Build history of the part. All positions in model axes, mm. Face numbers are marked on the shaded views. A direction names the side the tool comes from. Round coordinates to 2 decimals unless told otherwise and drop trailing zeros. Write each loop counter-clockwise with the first axis right and the second up, starting at its lowest first coordinate (ties: lowest second). Pieces come first, ordered by that corner, then holes. Notation, with made-up numbers: (1.5, 42.5) - (28.5, 42.5) arc R24 ccw to (28.5, 81.5) - close; hole circle Ø3 at (69, 58). An arc over 180 degrees is marked (long way). Write each question's results on one line, items separated by ' | '.
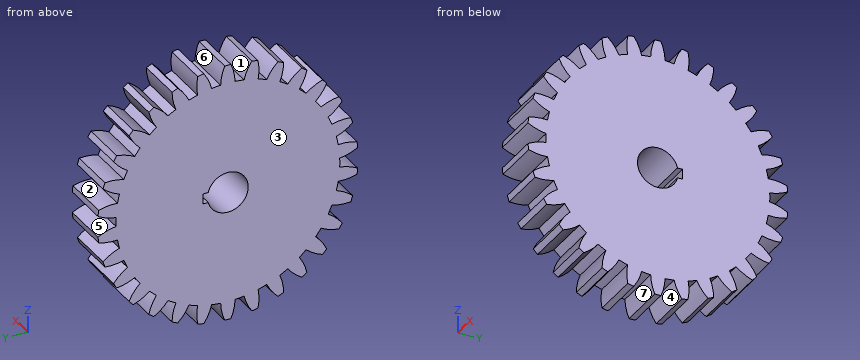
from build123d import *

# Parameters (mm, degrees)
BASPROSKE_W     = 304.8
BASPROSKE_H     = 812.8
TOOTHCUT_DEPTH  = 1190.197510929
TEETHCUTS_COUNT = 30
TEETHCUTS_ANGLE = 348
BORSKE_R        = 127
BORE_DEPTH      = 304.8000508
KEYSKE_W        = 63.5
KEYSKE_H        = 154.8384
KEYWAY_DEPTH    = 304.8000508


with BuildPart() as part:
    # BasProSke → Base-Revolve (revolve)
    with BuildSketch(Plane(origin=(0, 0, 0), x_dir=(1, 0, 0), z_dir=(0, 1, 0)), mode=Mode.PRIVATE) as base_revolve_sk:
        with Locations((152.4, 406.4)):
            Rectangle(BASPROSKE_W, BASPROSKE_H)
    revolve(base_revolve_sk.sketch.rotate(Axis((-10, 0, 0), (1, 0, 0)), 180), axis=Axis((-10, 0, 0), (1, 0, 0)))

    # TooCutSke → ToothCut (cut, through all)
    with BuildSketch(Plane(origin=(0, 0, 0), x_dir=(0, 0, -1), z_dir=(1, 0, 0))):
        with BuildLine():
            ThreePointArc((28.319737367, 697.924400123), (0, 698.49873), (-28.319737367, 697.924400123))
            ThreePointArc((-28.319737367, 697.924400123), (-41.533758507, 755.876600482), (-65.744032335, 810.162238751))
            ThreePointArc((-65.744032335, 810.162238751), (0, 812.8254), (65.744032335, 810.162238751))
            ThreePointArc((65.744032335, 810.162238751), (41.533758507, 755.876600482), (28.319737367, 697.924400123))
        make_face()
    toothcut = extrude(amount=TOOTHCUT_DEPTH, mode=Mode.SUBTRACT)

    # TeethCuts: ToothCut ×30 about axis
    teethcuts_axis = Axis((-10, 0, 0), (1, 0, 0))
    for i in range(1, TEETHCUTS_COUNT):
        add(toothcut.rotate(teethcuts_axis, i * TEETHCUTS_ANGLE / (TEETHCUTS_COUNT - 1)), mode=Mode.SUBTRACT)

    # BorSke → Bore (cut, symmetric)
    with BuildSketch(Plane(origin=(0, 0, 0), x_dir=(0, 0, -1), z_dir=(1, 0, 0))):
        with Locations(Location((0, 0, 0), (0, 0, 180))):
            Circle(BORSKE_R)
    extrude(amount=BORE_DEPTH, both=True, mode=Mode.SUBTRACT)

    # KeySke → Keyway (cut, symmetric)
    with BuildSketch(Plane(origin=(0, 0, 0), x_dir=(0, 0, -1), z_dir=(1, 0, 0))):
        with Locations((0, 77.4192)):
            Rectangle(KEYSKE_W, KEYSKE_H)
    extrude(amount=KEYWAY_DEPTH, both=True, mode=Mode.SUBTRACT)


solid = part.part
(1) Drill centre lines: probe 1 along Y at (x, z) = (173.5, 9); probe 2 along Y at (x, z) = (225.5, 0); probe 3 along Z at (x, y) = (63, 0). Where is each one in solid material? Low to high. Write a range as [from, to].
Worked answers:
probe 1: y = [-698.44, -126.68], [154.84, 698.44] | probe 2: y = [-698.5, -127], [154.84, 698.5] | probe 3: z = [-812.8, -127], [127, 812.8]
(2) Tool access for the marked faces 5, 6 and 7: list every direction of +Z, -Z, +X, -X, +Y, -Y with a clear straight run to the whole face (end or side of a thin tool).
Worked answers:
face 5: +X, -X, +Y | face 6: +Z, +X, -X | face 7: -Z, +X, -X
(3) Two-plate mould, pull along Z, no slides. Class the marked faces 1, 2, 3 and 4: released by +Z, released by -Z, zero draft, split by the parting line, or undercut.
Worked answers:
face 1: released by +Z | face 2: undercut | face 3: zero draft | face 4: released by -Z
(4) Slice it at A-A, the plane z = 0. Write the cut outline in (x, y).
Worked answers:
outline: (0, -698.5) - (304.8, -698.5) - (304.8, -127) - (0, -127) - close; (0, 154.84) - (304.8, 154.84) - (304.8, 698.5) - (0, 698.5) - close
(5) Slice it at C-C, the plane y = 274.5. Write the cut outline in (x, z).
Worked answers:
outline: (0, -707.95) - (304.8, -707.95) - (304.8, 707.95) - (0, 707.95) - close
(6) Flat gauge pins, fed straight in: pin 1 Ø1 at (x, y) = (253.5, 301.5) entering from -Z; pin 2 Ø1.5 at (x, y) = (36, -129) entering from +Z; pin 3 Ø2 at (x, z) = (142.5, -615.5) entering from -Y. Where does each tip first touch, or does it go through?
Worked answers:
pin 1: stops at z = -739.77 | pin 2: stops at z = 766.37 | pin 3: stops at y = -485.19
(7) Slice it at B-B, the plane y = 0. Write the cut outline in (x, z), and give its area (3 significant figures).
Worked answers:
outline: (0, -812.8) - (304.8, -812.8) - (304.8, -127) - (0, -127) - close; (0, 127) - (304.8, 127) - (304.8, 812.8) - (0, 812.8) - close | area: 418,000 mm2
